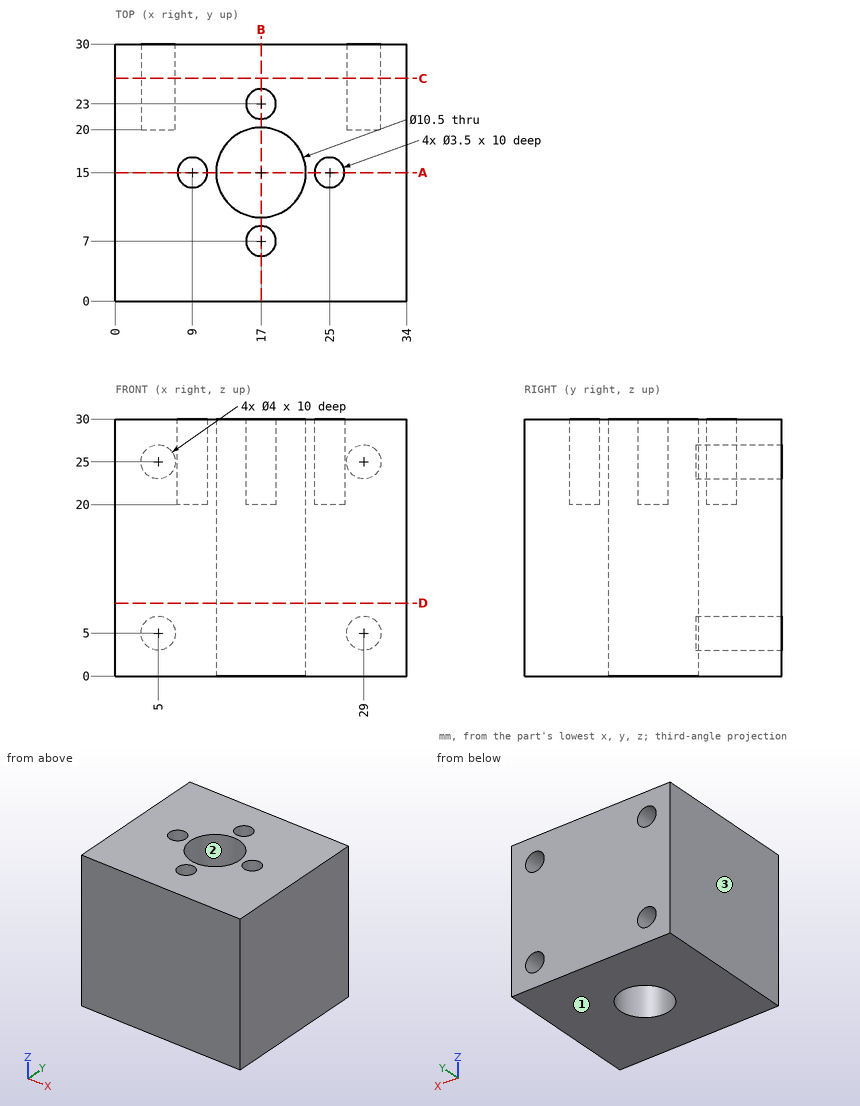
Job drawing, mm, ordinate dimensions from the low corner. One solid piece. Round coordinates to 2 decimals unless told otherwise and drop trailing zeros. Write each loop counter-clockwise with the first axis right and the second up, starting at its lowest first coordinate (ties: lowest second). Pieces come first, ordered by that corner, then holes. Notation, with made-up numbers: (-19.5, 67) -> (26.5, 67) arc R17 ccw to (26.5, 93) -> close; hole circle Ø7 at (32, 38.25). An arc over 180 degrees is marked (long way). Answer as a JSON object with one key per item and string values.
(1) Probe probe 1 along Y at (x, z) = (17, 26); probe 2 along Z at (x, y) = (5, 22.75); probe 3 along Y at (x, z) = (25, 23). List the from-to ranges inside material, lowest first. Write a range as [from, to].
Reported:
{"probe 1": "y = [0, 5.25], [8.75, 9.75], [20.25, 21.25], [24.75, 30]", "probe 2": "z = [0, 3], [7, 23], [27, 30]", "probe 3": "y = [0, 13.25], [16.75, 30]"}
(2) Band-saw the part on B-B, the plane x = 17. List the corners of the cut face in (y, z), then the cut area to 3 significant figures.
Reported:
{"outline": "(0, 0) -> (9.75, 0) -> (9.75, 30) -> (8.75, 30) -> (8.75, 20) -> (5.25, 20) -> (5.25, 30) -> (0, 30) -> close; (20.25, 0) -> (30, 0) -> (30, 30) -> (24.75, 30) -> (24.75, 20) -> (21.25, 20) -> (21.25, 30) -> (20.25, 30) -> close", "area": "515 mm^2"}
(3) Band-saw the part on A-A, the plane y = 15. List the corners of the cut face in (x, z).
Reported:
{"outline": "(0, 0) -> (11.75, 0) -> (11.75, 30) -> (10.75, 30) -> (10.75, 20) -> (7.25, 20) -> (7.25, 30) -> (0, 30) -> close; (22.25, 0) -> (34, 0) -> (34, 30) -> (26.75, 30) -> (26.75, 20) -> (23.25, 20) -> (23.25, 30) -> (22.25, 30) -> close"}
(4) Band-saw the part on D-D, the plane z = 8.5. List the corners of the cut face in (x, y), then the cut area to 3 significant figures.
Reported:
{"outline": "(0, 0) -> (34, 0) -> (34, 30) -> (0, 30) -> close; hole circle Ø10.5 at (17, 15)", "area": "933 mm^2"}
(5) Two-plate mould, pull along X, no slides. Class the marked faces 1, 2 and 3: +X half, -X half, draft (parallel to the pull), parting line (faces both ways), or undercut.
Reported:
{"face 1": "draft", "face 2": "undercut", "face 3": "-X half"}
(6) Pin check, flat tips, straight feed: P1, Ø4.5, axis at x = 28.5, z = 4, coming from the +Y side; P2, Ø2, axis at x = 25, y = 15, coming from the +Z side; P3, Ø1.2, axis at x = 28.5, z = 24.5, coming from the +Y side. Stop position of each tip, or through.
Reported:
{"P1": "stops at y = 30", "P2": "stops at z = 20", "P3": "stops at y = 20"}
(7) Band-saw the part on C-C, the plane y = 26. List the corners of the cut face in (x, z).
Reported:
{"outline": "(0, 0) -> (34, 0) -> (34, 30) -> (0, 30) -> close; hole circle Ø4 at (5, 5); hole circle Ø4 at (5, 25); hole circle Ø4 at (29, 5); hole circle Ø4 at (29, 25)"}
